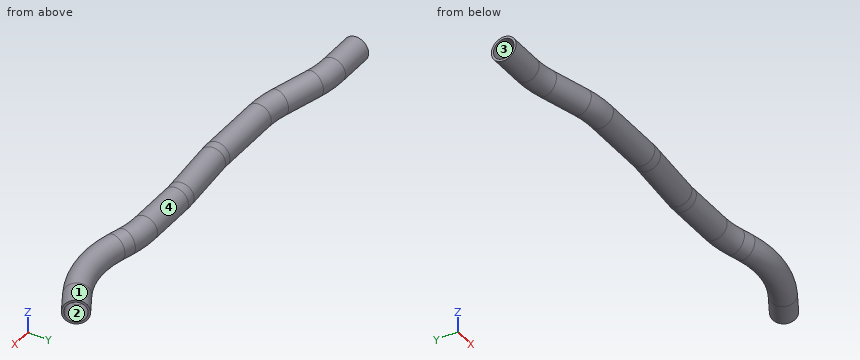
from build123d import *

# Parameters (mm, degrees)
SKETCH2_R   = 9.525
SKETCH2_R_2 = 7.874


with BuildPart() as part:
    # Sweep1: sweep along a path in Sketch1
    with BuildLine(Plane.XY) as sweep1_path:
        Line((124.181687085, -15.949323606), (152.249766769, -15.949323606))
        ThreePointArc((152.249766769, -15.949323606), (162.195862616, -16.601225169), (171.971778005, -18.545775643))
        Line((171.971778005, -18.545775643), (201.66062814, -26.50087906))
        ThreePointArc((201.66062814, -26.50087906), (211.436543529, -28.445429534), (221.382639376, -29.097331097))
        Line((221.382639376, -29.097331097), (271.523755211, -29.097331097))
        ThreePointArc((271.523755211, -29.097331097), (274.847552528, -29.024805582), (278.165022808, -28.807367092))
        Line((278.165022808, -28.807367092), (322.143105976, -24.959783371))
        ThreePointArc((322.143105976, -24.959783371), (325.460576256, -24.742344881), (328.784373573, -24.669819366))
        Line((328.784373573, -24.669819366), (366.225489407, -24.669819366))
        ThreePointArc((366.225489407, -24.669819366), (376.171585254, -25.321720929), (385.947500644, -27.266271402))
        Line((385.947500644, -27.266271402), (394.838853894, -29.648702325))
        ThreePointArc((394.838853894, -29.648702325), (424.506960978, -31.593252799), (452.66086513, -22.03629013))
        Line((452.66086513, -22.03629013), (469.320532211, -12.417826857))
    # Sketch2 → Sweep1 (sweep)
    with BuildSketch(Plane(origin=(124.181687085, -15.949323606, 0), x_dir=(0, 0, -1), z_dir=(1, 0, 0))):
        Circle(SKETCH2_R)
        Circle(SKETCH2_R_2, mode=Mode.SUBTRACT)
    sweep(path=sweep1_path.line)


solid = part.part
Read the model definition and answer for the solid it produces. Units are mm, in the model's axes. Face numbers are marked on the shaded views. A direction names the side the tool comes from. Coordinates: 2 decimals unless noted, no trailing zeros. Write each loop counter-clockwise with the first axis right and the second up, starting at its lowest first coordinate (ties: lowest second). Pieces come first, ordered by that corner, then holes. Notation, with made-up numbers: (59.5, 10.5) -> (100.5, 10.5) arc R8 ccw to (100.5, 14.5) -> close; hole circle Ø3 at (-38.75, -36.75). An arc over 180 degrees is marked (long way). Return JSON: item names as keys, results as strings.
(1) Each of these flat-tipped pins is pushed along its axis until it touches: P1, Ø2, axis at x = 180, z = 2, coming from the +Y side; P2, Ø1.5, axis at y = -17.5, z = -4.5, coming from the +X side; P3, Ø8, axis at y = -34.5, z = 7.5, coming from the +X side. Where does it stop, or does it pass through?
Answers below:
{"P1": "y = -10.73", "P2": "x = 472.69", "P3": "x = 452.43"}
(2) The part is cut by section A-A on x = 229.5. Give the vertices of the cut face in (y, z) (3 decimals).
Answers below:
{"outline": "circle Ø19.05 at (-29.097, 0); hole circle Ø15.748 at (-29.097, 0)"}
(3) Consider line 1 along Y through (x, z) = (134, 0); line 2 along Y through (x, z) = (249.5, 0); line 3 along Z through (x, y) = (376.5, -22). Determine where each line is inside the solid, lowest interval first. Write a range as from..to.
Answers below:
{"line 1": "-25.47..-23.82, -8.08..-6.42", "line 2": "-38.62..-36.97, -21.22..-19.57", "line 3": "-8.92..-7.13, 7.13..8.92"}
(4) Which of the six approach directions +Z, -Z, +X, -X, +Y, -Y give full straight-line access (tool end or side, diameter ignored) to the marked faces 3 and 4?
Answers below:
{"face 3": "-X", "face 4": "none"}
(5) For a pull along Z with two mould halves and no side action, classify the marked faces 1 and 2 as pulls with the +Z half, pulls with the -Z half, needs draft (parallel to the pull), parting line crosses it, or undercut.
Answers below:
{"face 1": "parting line crosses it", "face 2": "undercut"}
